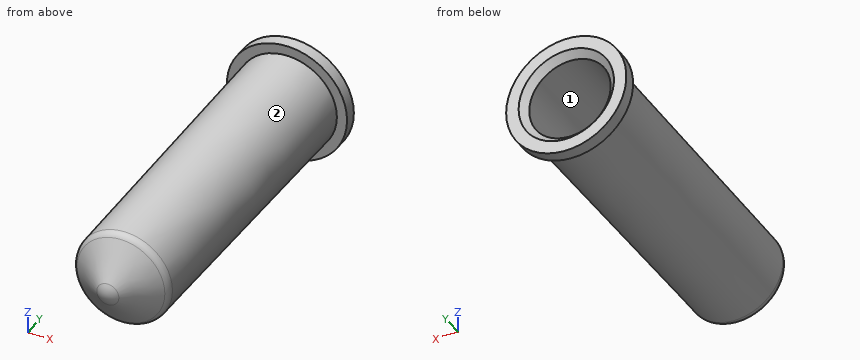
from build123d import *


with BuildPart() as part:
    # Sketch1 → Revolve1 (revolve)
    with BuildSketch(Plane.XY):
        with BuildLine():
            Line((1.197299905, -3.457984677), (4.752406997, -0.801010758))
            ThreePointArc((4.752406997, -0.801010758), (5.046117858, -0.451322699), (5.153728827, -0.007512281))
            Line((5.153728827, -0.007512281), (5.4, 32.774036839))
            Line((5.4, 32.774036839), (6.504629528, 32.774036839))
            Line((6.504629528, 32.774036839), (6.504629528, 34.144036839))
            Line((6.504629528, 34.144036839), (5.154629528, 34.144036839))
            Line((5.154629528, 34.144036839), (4.404629528, 33.394036839))
            Line((4.404629528, 33.394036839), (4.153757045, 0))
            Line((4.153757045, 0), (0.598649953, -2.656973919))
            ThreePointArc((0.598649953, -2.656973919), (0.31542768, -2.80491278), (0, -2.855963161))
            Line((0, -2.855963161), (0, -3.855963161))
            ThreePointArc((0, -3.855963161), (0.630855359, -3.753862399), (1.197299905, -3.457984677))
        make_face()
    revolve(axis=Axis((0, 0, 0), (0, 1, 0)))


solid = part.part
Input: part model. Units: mm. Frame: model coordinates. Face numbers are marked on the shaded views. A direction names the side the tool comes from. Round coordinates to 2 decimals unless told otherwise and drop trailing zeros. Loops run counter-clockwise (first coordinate to the right, second up) from the corner with the lowest first, then second, coordinate; pieces in that order, holes last. Notation, with made-up numbers: (-38.75, 58) -> (-16.75, 58) arc R10 ccw to (-16.75, 70) -> close; hole circle Ø2 at (75.25, -30). An arc over 180 degrees is marked (long way). Answer as a JSON object with one key per item and string values. Group by question number.
1) Section query B-B on y = 6. Output: boundary loops of the cut face in (x, z), plus the area to 3 significant figures.
2) Pin query (flat end, axial travel): pin 1 (5 mm diameter, centred on x = 1, y = 30, fed in from +Z); pin 2 (3 mm diameter, centred on x = 3, y = 30, fed in from -Z); pin 3 (6 mm diameter, centred on y = 7.5, z = 1, fed in from -X). Return the tip coordinate at first contact, or that it passes through.
3) Ray query, L1, parallel to X at y = 16.5, z = -0.5; L2, parallel to Z at x = -2.5, y = 2; L3, parallel to X at y = 19, z = 3.25. Return the intervals inside material, ascending.
4) Section query A-A on y = 16. Output: boundary loops of the cut face in (x, z).
5) Reachability of the marked faces 1 and 2 from +Z, -Z, +X, -X, +Y, -Y: full face, straight path, thin tool, end or side. Return the list, or none.
Reply:
{
 "1": {"outline": "circle Ø10.4 at (0, 0); hole circle Ø8.4 at (0, 0)", "area": "29.5 mm2"},
 "2": {"pin 1": "stops at z = 5.4", "pin 2": "stops at z = -5.17", "pin 3": "stops at x = -5.23"},
 "3": {"L1": "x = -5.25 to -4.25, 4.25 to 5.25", "L2": "z = -4.52 to -3.34, 3.34 to 4.52", "L3": "x = -4.18 to -2.81, 2.81 to 4.18"},
 "4": {"outline": "circle Ø10.55 at (0, 0); hole circle Ø8.55 at (0, 0)"},
 "5": {"face 1": "+Y", "face 2": "-Y"}
}
